Autodesk Fusion 360 part; units mm, degrees
sketch "Sketch1" plane through (0, 0, 0) normal (0, 0, 1) x (1, 0, 0)
  line L0 (-22.5, 22.5) -> (22.5, 22.5)
  line L1 (22.5, 22.5) -> (22.5, -22.5)
  line L2 (22.5, -22.5) -> (-22.5, -22.5)
  line L3 (-22.5, -22.5) -> (-22.5, 22.5)
  line L4 (-22.5, 22.5) -> (22.5, -22.5) construction
  line L5 (22.5, 22.5) -> (-22.5, -22.5) construction
  circle A0 centre (-15, 15) radius 1.25
  circle A1 centre (15, 15) radius 1.25
  circle A2 centre (15, -15) radius 1.25
  circle A3 centre (-15, -15) radius 1.25
  line L6 (-30, 30) -> (30, 30)
  line L7 (30, 30) -> (30, -30)
  line L8 (30, -30) -> (-30, -30)
  line L9 (-30, -30) -> (-30, 30)
  line L10 (-30, 30) -> (30, -30) construction
  line L11 (30, 30) -> (-30, -30) construction
  line L12 (-12.5, -22.5) -> (12.5, -22.5)
  line L13 (12.5, -22.5) -> (12.5, -30)
  line L14 (12.5, -30) -> (-12.5, -30)
  line L15 (-12.5, -30) -> (-12.5, -22.5)
  dimension "d1" = 45
  dimension "d2" = 45
  dimension "d3" = 2.5
  dimension "d4" = 2.5
  dimension "d5" = 2.5
  dimension "d6" = 2.5
  dimension "d7" = 7.5
  dimension "d9" = 7.5
  dimension "d10" = 7.5
  dimension "d11" = 7.5
  dimension "d12" = 60
  dimension "d13" = 60
  dimension "d14" = 7.5
  dimension "d15" = 10
  dimension "d16" = 10
extrude "Extrude1" add sketch "Sketch1" along normal blind 22 contours L0 L1 L2 L3 L6 L7 L8 L9 L13 L15
extrude "Extrude2" add sketch "Sketch1" along normal blind 2 contours L0 L1 L2 L3 L12
extrude "Extrude3" add sketch "Sketch1" along normal blind 2 contours L2 L8 L12 L13 L14 L15
sketch "Sketch2" plane through (0, 0, 22) normal (0, 0, 1) x (1, 0, 0)
  line L0 (-30, -30) -> (-12.5, -30)
  line L1 (-12.5, -30) -> (-12.5, -22.5)
  line L2 (-12.5, -22.5) -> (-22.5, -22.5)
  line L3 (-22.5, -22.5) -> (-22.5, 22.5)
  line L4 (-22.5, 22.5) -> (22.5, 22.5)
  line L5 (22.5, 22.5) -> (22.5, -22.5)
  line L6 (22.5, -22.5) -> (12.5, -22.5)
  line L7 (12.5, -22.5) -> (12.5, -30)
  line L8 (12.5, -30) -> (30, -30)
  line L9 (30, -30) -> (30, 30)
  line L10 (30, 30) -> (-30, 30)
  line L11 (-30, 30) -> (-30, -30)
  circle A0 centre (-25.75, 25.75) radius 2
  circle A1 centre (25.75, 25.75) radius 2
  circle A2 centre (-25.75, -25.75) radius 2
  circle A3 centre (25.75, -25.75) radius 2
  dimension "d23" = 4
  dimension "d24" = 4.25
  dimension "d25" = 4.25
  dimension "d26" = 4
  dimension "d27" = 4.25
  dimension "d28" = 4.25
  dimension "d29" = 4
  dimension "d30" = 4.25
  dimension "d31" = 4.25
  dimension "d32" = 4
  dimension "d33" = 4.25
  dimension "d34" = 4.25
extrude "Extrude4" cut sketch "Sketch2" against normal blind 4.72 contours A0 | A1 | A2 | A3
equation "d24 = holesfromcorner"
equation "d25 = holesfromcorner"
equation "d27 = holesfromcorner"
equation "d28 = holesfromcorner"
equation "d30 = holesfromcorner"
equation "d31 = holesfromcorner"
equation "d33 = holesfromcorner"
equation "d34 = holesfromcorner"
equation "holesfromcorner = 4.25 mm"
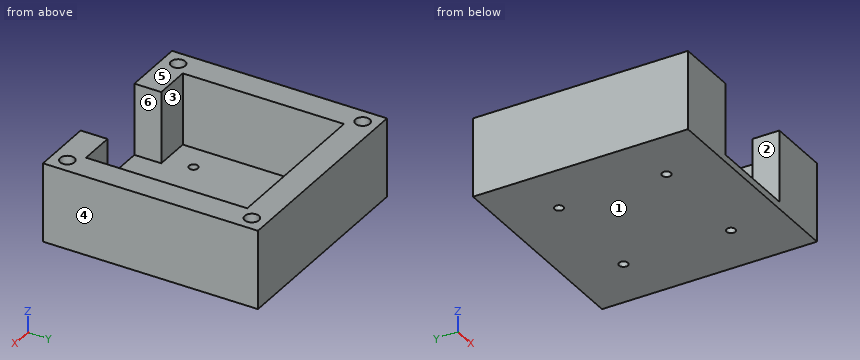
Part model, mm, in its own coordinate system. Face numbers are marked on the shaded views. A direction names the side the tool comes from. Round coordinates to 2 decimals unless told otherwise and drop trailing zeros. Write each loop counter-clockwise with the first axis right and the second up, starting at its lowest first coordinate (ties: lowest second). Pieces come first, ordered by that corner, then holes. Notation, with made-up numbers: (51, 6.5) - (82, 6.5) arc R19 cw to (82, 35.5) - close; hole circle Ø8 at (21, 66). An arc over 180 degrees is marked (long way). Use CSV: the item, a comma, the result in double quotes.
Item 1: Tool access for the marked faces 1, 2 and 3: list every direction of +Z, -Z, +X, -X, +Y, -Y with a clear straight run to the whole face (end or side of a thin tool).
Results list:
face 1,"-Z, +X, -X, +Y, -Y"
face 2,"+Z, -Y"
face 3,"+Z"
Item 2: Slice it at B-B, the plane z = 11.75. Write the cut outline in (x, y).
Results list:
outline,"(-30, -30) - (-12.5, -30) - (-12.5, -22.5) - (-22.5, -22.5) - (-22.5, 22.5) - (22.5, 22.5) - (22.5, -22.5) - (12.5, -22.5) - (12.5, -30) - (30, -30) - (30, 30) - (-30, 30) - close"
Item 3: Slice it at C-C, the plane x = -21. Write the cut outline in (y, z), then the cut area to 3 significant figures.
Results list:
outline,"(-30, 0) - (30, 0) - (30, 22) - (22.5, 22) - (22.5, 2) - (-22.5, 2) - (-22.5, 22) - (-30, 22) - close"
area,"420 mm²"
Item 4: Wall check: L1, parallel to Y at x = -25.75, z = 18.3; L2, parallel to Y at x = 15, z = 1.35; L3, parallel to X at y = -12.5, z = 17.5. Give the ranges that are in metal, low to high.
Results list:
L1,"y = -30 to -27.75, -23.75 to 23.75, 27.75 to 30"
L2,"y = -30 to -16.25, -13.75 to 13.75, 16.25 to 30"
L3,"x = -30 to -22.5, 22.5 to 30"
Item 5: Slice it at A-A, the plane y = -15. Write the cut outline in (x, z), then the cut area to 3 significant figures.
Results list:
outline,"(-30, 0) - (-16.25, 0) - (-16.25, 2) - (-22.5, 2) - (-22.5, 22) - (-30, 22) - close; (-13.75, 0) - (13.75, 0) - (13.75, 2) - (-13.75, 2) - close; (16.25, 0) - (30, 0) - (30, 22) - (22.5, 22) - (22.5, 2) - (16.25, 2) - close"
area,"410 mm²"
Item 6: Flat gauge pin, fed straight in: P1, Ø3, axis at x = 15, y = 15, coming from the +Z side. Where does the tip first touch, or does it go through?
Results list:
P1,"stops at z = 2"
Item 7: Pull direction X, two halves, no side cores. Call the marked faces 4, 5 and 6: pulls with the +X half, pulls with the -X half, needs draft (parallel to the pull), parting line crosses it, or undercut.
Results list:
face 4,"pulls with the +X half"
face 5,"needs draft"
face 6,"undercut"
